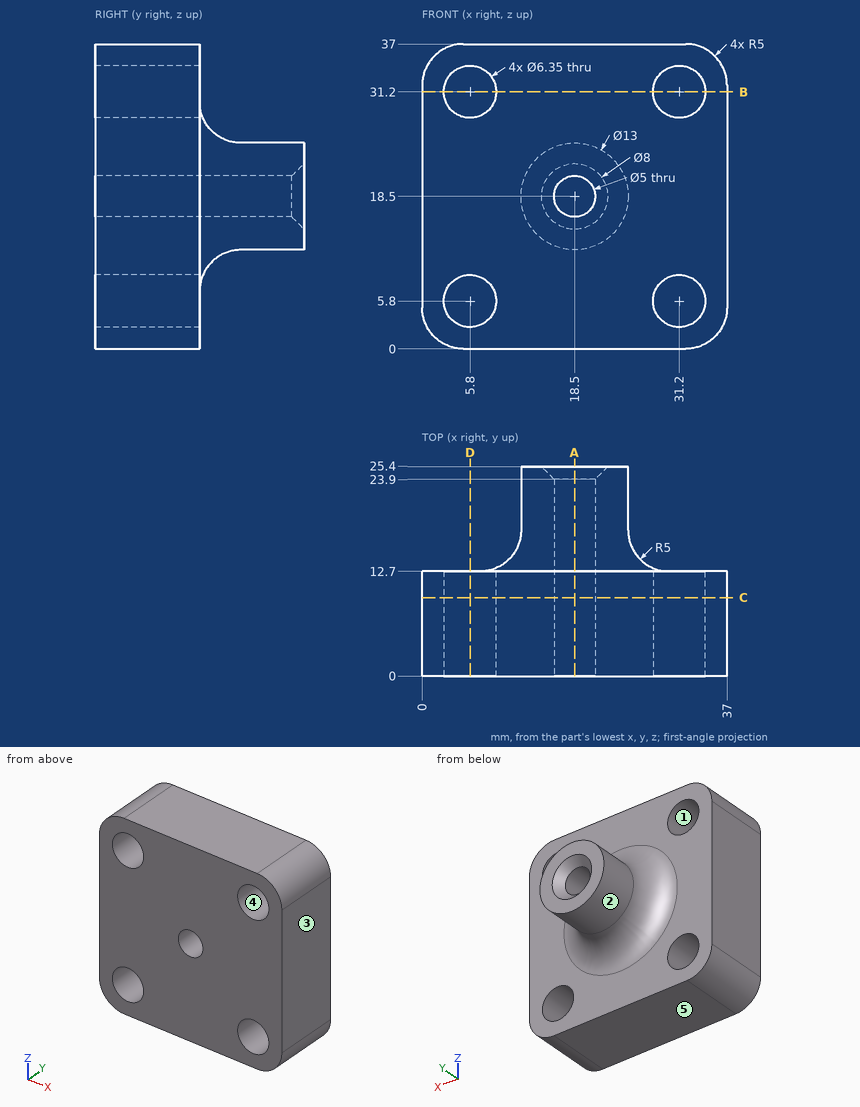
Input: dimensioned drawing with shaded views. Units: mm. Origin: part minimum x, y, z. A direction names the side the tool comes from. Coordinates: 2 decimals unless noted, no trailing zeros. Order: outer loops, then holes, each group sorted by start corner. A loop starts at its lowest first (then second) coordinate and runs counter-clockwise, first axis right, second up. Notation, with made-up numbers: (25.5, 60.5) -> (42.5, 60.5) arc R14 cw to (42.5, 87.5) -> close; hole circle Ø4 at (76, 42). An arc over 180 degrees is marked (long way). Answer in a Markdown table with one row per item.
Item 1: Contact query for flat-ended pins moving along their axis: P1, Ø12, axis at x = 4.5, y = 7.5, coming from the -Z side; P2, Ø12, axis at x = 32.5, y = 20, coming from the -Z side; P3, Ø5, axis at x = 10.5, z = 24.5, coming from the +Y side; P4, Ø3, axis at x = 28, z = 29.5, coming from the +Y side. Output: stop coordinate, or through.
Return value:
| item | result |
|---|---|
| P1 | stops at z = 0 |
| P2 | passes through |
| P3 | stops at y = 14.7 |
| P4 | stops at y = 12.7 |
Item 2: Draft query along X for the marked faces 3, 4 and 5. Return one class per face: released by +X, released by -X, zero draft, split by the parting line, or undercut.
Return value:
| item | result |
|---|---|
| face 3 | released by +X |
| face 4 | undercut |
| face 5 | zero draft |
Item 3: Section A-A on x = 18.5. Output: boundary loops of the cut face in (y, z).
Return value:
| item | result |
|---|---|
| outline | (0, 0) -> (12.7, 0) -> (12.7, 7) arc R5 cw to (17.7, 12) -> (25.4, 12) -> (25.4, 14.5) -> (23.9, 16) -> (0, 16) -> close; (0, 21) -> (23.9, 21) -> (25.4, 22.5) -> (25.4, 25) -> (17.7, 25) arc R5 cw to (12.7, 30) -> (12.7, 37) -> (0, 37) -> close |
Item 4: Section C-C on y = 9.5. Output: boundary loops of the cut face in (x, z) (3 decimals).
Return value:
| item | result |
|---|---|
| outline | (0, 5) arc R5 ccw to (5, 0) -> (32, 0) arc R5 ccw to (37, 5) -> (37, 32) arc R5 ccw to (32, 37) -> (5, 37) arc R5 ccw to (0, 32) -> close; hole circle Ø6.35 at (5.8, 5.8); hole circle Ø6.35 at (5.8, 31.2); hole circle Ø5 at (18.5, 18.5); hole circle Ø6.35 at (31.2, 5.8); hole circle Ø6.35 at (31.2, 31.2) |
Item 5: Section B-B on z = 31.2. Output: boundary loops of the cut face in (x, y) (3 decimals).
Return value:
| item | result |
|---|---|
| outline | (0, 0) -> (2.625, 0) -> (2.625, 12.7) -> (0, 12.7) -> close; (8.975, 0) -> (28.025, 0) -> (28.025, 12.7) -> (8.975, 12.7) -> close; (34.375, 0) -> (37, 0) -> (37, 12.7) -> (34.375, 12.7) -> close |
Item 6: Access query for the marked faces 1 and 2. Directions: +Z, -Z, +X, -X, +Y, -Y. A direction counts if a zero-diameter tool reaches every point of the face in a straight line with its end or side. Return the directions, or none.
Return value:
| item | result |
|---|---|
| face 1 | +Y, -Y |
| face 2 | +Y |
Item 7: Section D-D on x = 5.8. Output: boundary loops of the cut face in (y, z) (3 decimals), plus the area to 3 significant figures.
Return value:
| item | result |
|---|---|
| outline | (0, 0) -> (12.7, 0) -> (12.7, 2.625) -> (0, 2.625) -> close; (0, 8.975) -> (12.7, 8.975) -> (12.7, 28.025) -> (0, 28.025) -> close; (0, 34.375) -> (12.7, 34.375) -> (12.7, 37) -> (0, 37) -> close |
| area | 309 mm² |
Item 8: Ray query, L1, parallel to Z at x = 6, y = 5.25; L2, parallel to X at y = 6.5, z = 31.2 (3 decimals); L3, parallel to X at y = 11.5, z = 18.5. Return the intervals inside material, ascending.
Return value:
| item | result |
|---|---|
| L1 | z = 0 to 2.63, 8.97 to 28.03, 34.37 to 37 |
| L2 | x = 0 to 2.625, 8.975 to 28.025, 34.375 to 37 |
| L3 | x = 0 to 16, 21 to 37 |
